Geometry check sheet. Reference: the model listing, model coordinates, mm. Face numbers are marked on the shaded views. A direction names the side the tool comes from. Round coordinates to 2 decimals unless told otherwise and drop trailing zeros. Order: outer loops, then holes, each group sorted by start corner. A loop starts at its lowest first (then second) coordinate and runs counter-clockwise, first axis right, second up. Notation, with made-up numbers: (-17.75, 69) - (8.25, 69) arc R25 ccw to (8.25, 96) - close; hole circle Ø6 at (6.25, 50). An arc over 180 degrees is marked (long way). Return JSON: item names as keys, results as strings. Group by question number.
Q1. Tool access check on the marked faces 1 and 2. Record the directions out of +Z, -Z, +X, -X, +Y, -Y that give a thin tool (end or side, any length) a straight path to the whole face; none if there is none.
Q2. Sectioned sample at C-C, the plane y = 2. Give the number of separate pieces and of enclosed holes in the cut face, then the cut area to 3 significant figures.
Q3. Gauge pin test, flat ends, axial feed: pin 1 Ø5.5 at (x, z) = (-35.28, -44.55) entering from +Y; pin 2 Ø4 at (y, z) = (5.5, -22.5) entering from +X; pin 3 Ø3 at (x, y) = (-8.5, 9.5) entering from +Z; pin 4 Ø3 at (x, z) = (-35.28, 24.45) entering from -Y. Record the tip position at first contact, or that the pin passes through.
Q4. Sectioned sample at B-B, the plane y = 7.25. Record the cut outline in (x, z), then the cut area to 3 significant figures.
Q5. Material ranges on line 1 along X through (y, z) = (13.75, -32); line 2 along Z through (x, y) = (-35.5, 11.5); line 3 along X through (y, z) = (11.75, -44.5), recorded low to high.
Q6. Sectioned sample at A-A, the plane z = 10. Record the cut outline in (x, y), then the cut area to 3 significant figures.
```python
from build123d import *

# Parameters (mm, degrees)
SKETCH1_R           = 1.66
BOSS_EXTRUDE1_DEPTH = 15
CHAMFER1_SIZE       = 40
CHAMFER1_SIZE2      = 5.266099903
FILLET1_R           = 5
FILLET2_R           = 3


with BuildPart() as part:
    # Sketch1 → Boss-Extrude1 (new body)
    with BuildSketch(Plane(origin=(0, 0, 0), x_dir=(1, 0, 0), z_dir=(0, 1, 0))):
        Polygon((-40.27740406, 58.046693319), (-40.27740406, -28.953306681), (-30.27740406, -28.953306681), (-30.27740406, 51.046693319), (12.22259594, 51.046693319), (12.22259594, 58.046693319), align=None)
        with Locations(Location((-35.27740406, -24.453306681, 0), (0, 0, 270))):  # turned: the seam where the file's is
            Circle(SKETCH1_R, mode=Mode.SUBTRACT)
        with Locations(Location((-35.27740406, 44.546693319, 0), (0, 0, 270))):  # turned: the seam where the file's is
            Circle(SKETCH1_R, mode=Mode.SUBTRACT)
    extrude(amount=BOSS_EXTRUDE1_DEPTH)

    # Chamfer1
    chamfer1_edges = [part.edges().sort_by_distance(p)[0] for p in [
        (-40.27740406, 7.5, -58.046693319),
    ]]
    chamfer1_side = [part.faces().sort_by_distance(p)[0] for p in [
        (-14.02740406, 7.5, -58.046693319),
    ]]
    chamfer(chamfer1_edges, length=CHAMFER1_SIZE, length2=CHAMFER1_SIZE2, reference=chamfer1_side[0])

    # Fillet1
    fillet1_edges = [part.edges().sort_by_distance(p)[0] for p in [
        (-40.27740406, 7.5, -52.780593416),
    ]]
    fillet(fillet1_edges, radius=FILLET1_R)

    # Fillet2
    fillet2_edges = [part.edges().sort_by_distance(p)[0] for p in [
        (-40.27740406, 0, -9.72120221),
        (-18.10371954, 0, -55.699814363),
        (-39.036603097, 0, -51.692440176),
        (5.97259594, 0, -58.046693319),
    ]]
    fillet(fillet2_edges, radius=FILLET2_R)


solid = part.part
```
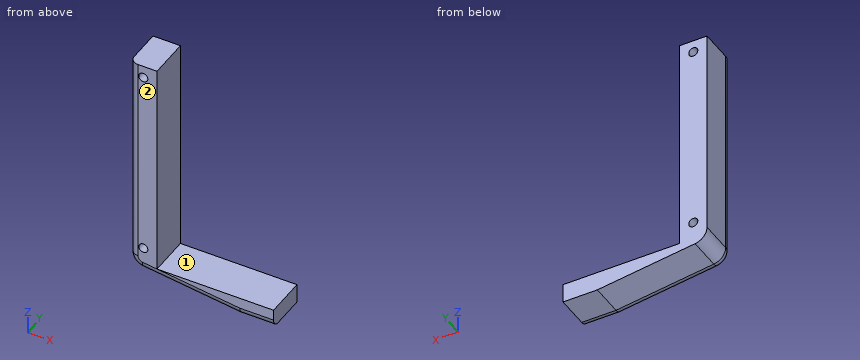
Reply:
{
 "1": {"face 1": "+Z, +X, +Y, -Y", "face 2": "+Z, -Z, +X, -X, -Y"},
 "2": {"separate pieces": "1", "enclosed holes": "2", "area": "1,020 mm^2"},
 "3": {"pin 1": "y = 15", "pin 2": "x = -30.28", "pin 3": "z = -51.05", "pin 4": "through"},
 "4": {"outline": "(-40.28, -48.4) arc R5 ccw to (-35.93, -53.35) - (-0.28, -58.05) - (12.22, -58.05) - (12.22, -51.05) - (-30.28, -51.05) - (-30.28, 28.95) - (-40.28, 28.95) - close; hole circle Ø3.32 at (-35.28, -44.55); hole circle Ø3.32 at (-35.28, 24.45)", "area": "1,040 mm^2"},
 "5": {"line 1": "-40.28 to -30.28", "line 2": "-53.41 to -46.19, -42.9 to 22.81, 26.1 to 28.95", "line 3": "-40.28 to -36.94, -33.62 to -30.28"},
 "6": {"outline": "(-40.28, 3) arc R3 ccw to (-37.28, 0) - (-30.28, 0) - (-30.28, 15) - (-40.28, 15) - close", "area": "148 mm^2"}
}
